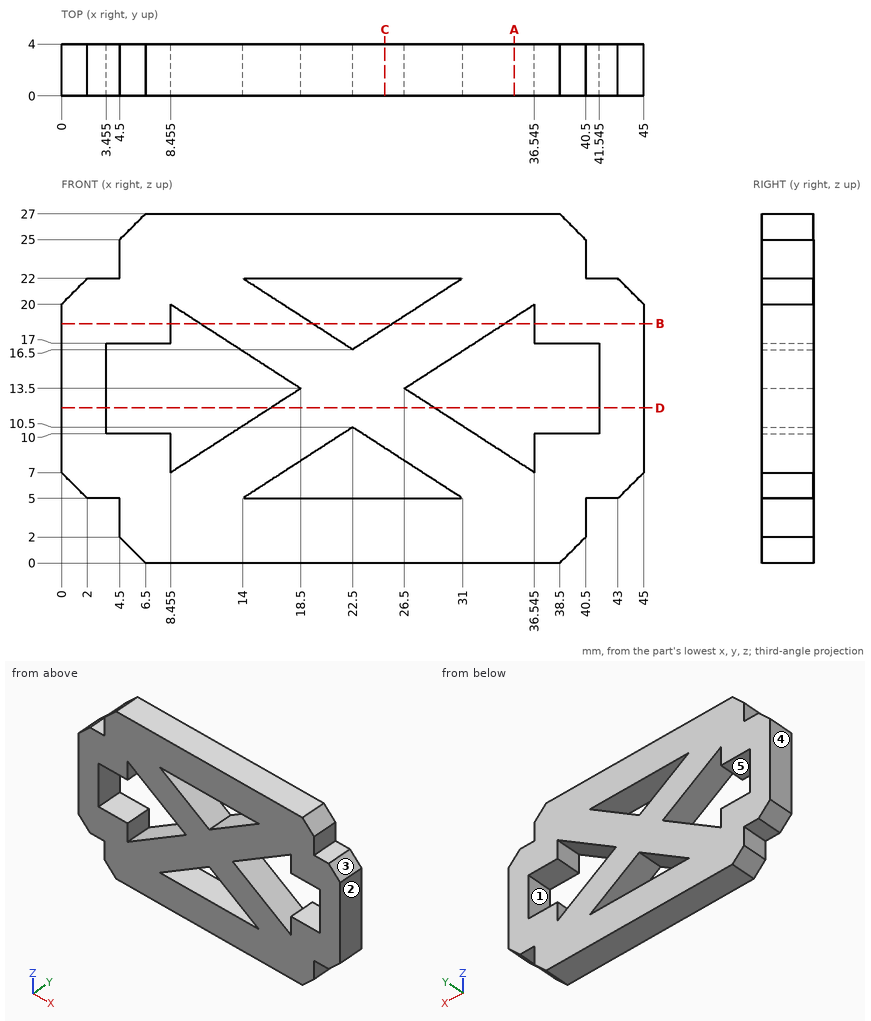
Here's the drawing with two shaded views (mm, measured from the low corner). I have some questions. A direction names the side the tool comes from. Coordinates: 2 decimals unless noted, no trailing zeros. Loops run counter-clockwise (first coordinate to the right, second up) from the corner with the lowest first, then second, coordinate; pieces in that order, holes last. Notation, with made-up numbers: (29.5, -4) -> (69.5, -4) arc R16 ccw to (69.5, 19) -> close; hole circle Ø11 at (-3.5, 39.25). An arc over 180 degrees is marked (long way). Put each result on its own line as item: value. Start each with the question number.
Q1. I want a section at C-C (x = 25). Write out the boundary of the cut face in (y, z).
Q2. I'm going to push flat-ended pins straight in: P1, Ø1.5, axis at y = 2, z = 3.5, coming from the +X side; P2, Ø0.8, axis at x = 4, y = 2.5, coming from the -Z side; P3, Ø1.5, axis at y = 1.5, z = 3.5, coming from the -X side. Where does each tip first touch, or does it pass through?
Q3. I want a section at B-B (z = 18.5). Write out the boundary of the cut face in (x, y) (1 decimal), plus the area to 3 significant figures.
Q4. I want a section at D-D (z = 12). Write out the boundary of the cut face in (x, y) (1 decimal).
Q5. I want a section at A-A (x = 35). Write out the boundary of the cut face in (y, z), plus the area to 3 significant figures.
Q6. For the marked faces 1 and 2, which set-ups out of +Z, -Z, +X, -X, +Y, -Y let a thin tool reach every point of the face, with its end or its side?
Q7. If I drill on line 1 (Z direction, x = 15, y = 0.6) (1 decimal); line 2 (X direction, y = 0.6, z = 13.75) (1 decimal); line 3 (Z direction, x = 24.5, y = 1.4) (1 decimal), over which ranges is the centre line in solid material (lowest first)? Write a range as [from, to].
Q8. Thinking about a two-plate mould opening in Z: for the marked faces 3, 4 and 5, which applies, pulls with the +Z half, pulls with the -Z half, needs draft (parallel to the pull), parting line crosses it, or undercut?
Taken from the geometry:
1. outline: (0, 0) -> (4, 0) -> (4, 5) -> (0, 5) -> close; (0, 8.88) -> (4, 8.88) -> (4, 18.12) -> (0, 18.12) -> close; (0, 22) -> (4, 22) -> (4, 27) -> (0, 27) -> close
2. P1: stops at x = 40.5
2. P2: stops at z = 5
2. P3: stops at x = 4.5
3. outline: (0, 0) -> (8.5, 0) -> (8.5, 4) -> (0, 4) -> close; (10.8, 0) -> (19.4, 0) -> (19.4, 4) -> (10.8, 4) -> close; (25.6, 0) -> (34.2, 0) -> (34.2, 4) -> (25.6, 4) -> close; (36.5, 0) -> (45, 0) -> (45, 4) -> (36.5, 4) -> close
3. area: 137 mm2
4. outline: (0, 0) -> (3.5, 0) -> (3.5, 4) -> (0, 4) -> close; (16.2, 0) -> (28.8, 0) -> (28.8, 4) -> (16.2, 4) -> close; (41.5, 0) -> (45, 0) -> (45, 4) -> (41.5, 4) -> close
5. outline: (0, 0) -> (4, 0) -> (4, 8) -> (0, 8) -> close; (0, 19) -> (4, 19) -> (4, 27) -> (0, 27) -> close
5. area: 64.0 mm2
6. face 1: +Y, -Y
6. face 2: +Z, -Z, +X, +Y, -Y
7. line 1: z = [0, 5], [5.6, 11.2], [15.8, 21.4], [22, 27]
7. line 2: x = [0, 3.5], [18.1, 26.9], [41.5, 45]
7. line 3: z = [0, 5], [9.2, 17.8], [22, 27]
8. face 3: pulls with the +Z half
8. face 4: needs draft
8. face 5: undercut
